Autodesk Inventor part; units mm, degrees
ref_plane "YZ Plane" through (0, 0, 0) normal (1, 0, 0) x (0, 1, 0)
ref_plane "XZ Plane" through (0, 0, 0) normal (0, 1, 0) x (-1, 0, 0)
ref_plane "XY Plane" through (0, 0, 0) normal (0, 0, 1) x (1, 0, 0)
sketch "Sketch5" plane through (0, 0, 0) normal (0, 1, 0) x (-1, 0, 0)
  line L0 (0, 0) -> (108, 0)
  line L1 (108, 0) -> (108, -130)
  line L2 (108, -130) -> (0, -130)
  line L3 (0, -130) -> (0, 0)
  dimension "d16" = 108
  dimension "d17" = 130
extrude "Extrusion4" add sketch "Sketch5" along normal blind 6
sketch "Sketch7" plane through (-108, 0, 0) normal (0, 0, 1) x (1, 0, 0)
  line L0 (0, 0) -> (108, 0)
  line L1 (108, 0) -> (108, 6)
  line L2 (0, 6) -> (108, 6)
  line L3 (0, 0) -> (0, 6)
  line L4 (108, 6) -> (0, 6)
  line L5 (0, 6) -> (0, 3)
  line L6 (108, 4) -> (108, 6)
  line L7 (108, 3) -> (0, 3)
  dimension "d35" = 3
extrude "Extrusion6" add sketch "Sketch7" along normal blind 2 and the other way blind 132 contours L3 L2 L1 L7
sketch "Sketch8" plane through (0, 0, 0) normal (1, 0, 0) x (0, 0, -1)
  line L0 (0, 0) -> (0, 3)
  line L1 (0, 0) -> (130, 0)
  line L2 (130, 0) -> (130, 3)
  line L3 (130, 3) -> (132, 3)
  line L4 (132, 6) -> (-2, 6)
  line L5 (-2, 3) -> (-2, 6)
  line L6 (0, 3) -> (130, 3)
  line L7 (132, 6) -> (132, 3)
  line L8 (-2, 3) -> (0, 3)
extrude "Extrusion7" add sketch "Sketch8" along normal blind 2 contours L8 L5 L4 L7 L3 L6
properties part number "TAPITA LA REAL AHORA SI"
Could you check a few things on this model? Use its own coordinates, in mm. A direction names the side the tool comes from. Coordinates: 2 decimals unless noted, no trailing zeros. Order: outer loops, then holes, each group sorted by start corner. A loop starts at its lowest first (then second) coordinate and runs counter-clockwise, first axis right, second up. Notation, with made-up numbers: (46.5, 84.25) -> (58.5, 84.25) arc R16 cw to (58.5, 110.25) -> close; hole circle Ø9 at (8, 44). An arc over 180 degrees is marked (long way). One line per item, written item: value. Start each with the question number.
1) I'm going to push flat-ended pins straight in: pin 1 (2.5 mm diameter, centred on x = -30.5, y = 2, fed in from -Z); pin 2 (1.5 mm diameter, centred on y = 2, z = -63.5, fed in from +X); pin 3 (2 mm diameter, centred on x = -12, y = 1, fed in from -Z). Where does each tip first touch, or does it pass through?
2) Which directions (+Z, -Z, +X, -X, +Y, -Y) give clear straight access to the entire face, cutting with the end or side of a thin tool? Please do faces 1 (the flat face through (-53, 0, -64)), 2 (the flat face through (-54, 5, -132)), 3 (the flat face through (0, 1, -66)), 4 (the flat face through (-53, 1, 0)), 5 (the flat face through (-55, 1, -130)).
3) If I drill on L1, parallel to X at y = 2.4, z = -38.5; L2, parallel to Z at x = -54, y = 0.45, over which ranges is the centre line in solid material (lowest first)? Write a range as [from, to].
4) Imagine slicing it at A-A on y = 1.45. List the corners of the cut face in (x, z) for me.
Answer list:
1. pin 1: stops at z = -132
1. pin 2: stops at x = 0
1. pin 3: stops at z = -130
2. face 1: +Z, -Z, +X, -X, -Y
2. face 2: -Z, +X, -X, +Y, -Y
2. face 3: +Z, -Z, +X, -Y
2. face 4: +Z, +X, -X, -Y
2. face 5: -Z, +X, -X, -Y
3. L1: x = [-108, 0]
3. L2: z = [-130, 0]
4. outline: (-108, -130) -> (0, -130) -> (0, 0) -> (-108, 0) -> close
